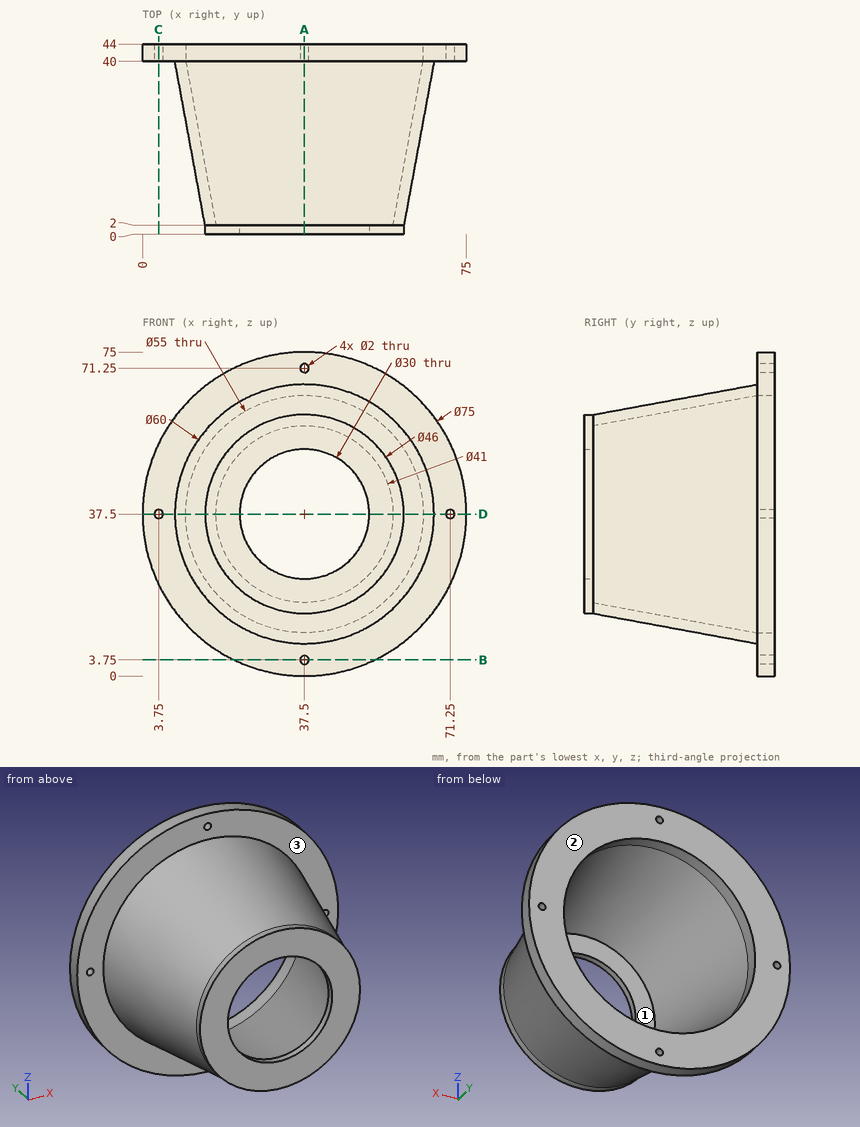
Geometry check sheet. Reference: drawing and pictorial views, mm from the part's lowest x, y, z. A direction names the side the tool comes from. Give positions to 0.01 mm unless a question says otherwise; leave off trailing zeros. Write each loop counter-clockwise with the first axis right and the second up, starting at its lowest first coordinate (ties: lowest second). Pieces come first, ordered by that corner, then holes. Notation, with made-up numbers: (68.25, 31.5) -> (73.25, 31.5) arc R24 ccw to (73.25, 55.5) -> close; hole circle Ø5 at (9.25, 85). An arc over 180 degrees is marked (long way). One line per item, written item: value. Start each with the question number.
Item 1: Section check B-B on z = 3.75. Record the cut outline in (x, y).
Item 2: Gauge pin test, flat ends, axial feed: pin 1 (1 mm diameter, centred on x = 21, z = 52.5, fed in from -Y); pin 2 (1.8 mm diameter, centred on x = 37.5, z = 3.75, fed in from +Y); pin 3 (2.5 mm diameter, centred on x = 37.5, z = 71.25, fed in from -Y); pin 4 (3 mm diameter, centred on x = 19.5, y = 17.5, fed in from -Z). Record the tip position at first contact, or that the pin passes through.
Item 3: Section check C-C on x = 3.75. Record the cut outline in (y, z), then the cut area to 3 significant figures.
Item 4: Tool access check on the marked faces 1, 2 and 3. Record the directions out of +Z, -Z, +X, -X, +Y, -Y that give a thin tool (end or side, any length) a straight path to the whole face; none if there is none.
Item 5: Section check A-A on x = 37.5. Record the cut outline in (y, z), then the cut area to 3 significant figures.
Item 6: Material ranges on probe 1 along Z at (x, y) = (37.5, 42.55); probe 2 along Z at (x, y) = (37, 1); probe 3 along Z at (x, y) = (37, 41), recorded low to high. Write a range as from..to.
Item 7: Section check D-D on z = 37.5. State how many separate pieces and enclosed holes the cut face has, then the cut area to 3 significant figures.
Results list:
1. outline: (21.15, 40) -> (36.5, 40) -> (36.5, 44) -> (21.15, 44) -> close; (38.5, 40) -> (53.85, 40) -> (53.85, 44) -> (38.5, 44) -> close
2. pin 1: y = 0
2. pin 2: through
2. pin 3: y = 40
2. pin 4: z = 17.54
3. outline: (40, 21.15) -> (44, 21.15) -> (44, 36.5) -> (40, 36.5) -> close; (40, 38.5) -> (44, 38.5) -> (44, 53.85) -> (40, 53.85) -> close
3. area: 123 mm²
4. face 1: +Y
4. face 2: +Z, -Z, +X, -X, +Y
4. face 3: -Y
5. outline: (0, 14.5) -> (2, 14.5) -> (40, 7.5) -> (40, 4.75) -> (44, 4.75) -> (44, 10) -> (40, 10) -> (2, 17) -> (2, 22.5) -> (0, 22.5) -> close; (0, 52.5) -> (2, 52.5) -> (2, 58) -> (40, 65) -> (44, 65) -> (44, 70.25) -> (40, 70.25) -> (40, 67.5) -> (2, 60.5) -> (0, 60.5) -> close; (40, 0) -> (44, 0) -> (44, 2.75) -> (40, 2.75) -> close; (40, 72.25) -> (44, 72.25) -> (44, 75) -> (40, 75) -> close
5. area: 286 mm²
6. probe 1: 0..2.75, 4.75..10, 65..70.25, 72.25..75
6. probe 2: 14.51..22.51, 52.49..60.49
6. probe 3: 0..2.88, 4.62..10, 65..70.38, 72.12..75
7. separate pieces: 4
7. enclosed holes: 0
7. area: 286 mm²
